Source: CAD feature listing. Evaluate the final solid. Frame: model axes, mm. Face numbers are marked on the shaded views. Coordinates: 2 decimals unless noted, no trailing zeros. Order: outer loops, then holes, each group sorted by start corner. A loop starts at its lowest first (then second) coordinate and runs counter-clockwise, first axis right, second up.
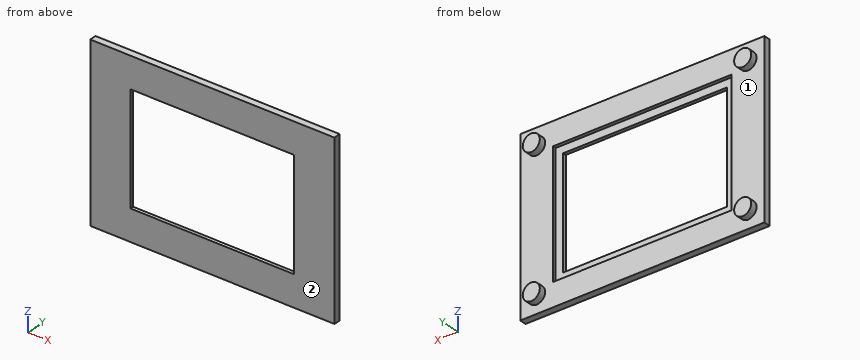
```python
from build123d import *

# Parameters (mm, degrees)
SKETCH1_W           = 35.8
SKETCH1_H           = 25
SKETCH1_W_2         = 24
SKETCH1_H_2         = 16
BOSS_EXTRUDE1_DEPTH = 1
SKETCH2_W           = 26.2
SKETCH2_H           = 18.2
CUT_EXTRUDE1_DEPTH  = 0.5
SKETCH4_R           = 1.25
BOSS_EXTRUDE2_DEPTH = 1


with BuildPart() as part:
    # Sketch1 → Boss-Extrude1 (new body)
    with BuildSketch(Plane(origin=(0, 0, 0), x_dir=(1, 0, 0), z_dir=(0, 1, 0))):
        Rectangle(SKETCH1_W, SKETCH1_H)
        Rectangle(SKETCH1_W_2, SKETCH1_H_2, mode=Mode.SUBTRACT)
    extrude(amount=BOSS_EXTRUDE1_DEPTH)

    # Sketch2 → Cut-Extrude1 (cut)
    with BuildSketch(Plane(origin=(0, 1, 0), x_dir=(1, 0, 0), z_dir=(0, 1, 0))):
        Rectangle(SKETCH2_W, SKETCH2_H)
    extrude(amount=-CUT_EXTRUDE1_DEPTH, mode=Mode.SUBTRACT)

    # Sketch4 → Boss-Extrude2 (add)
    with BuildSketch(Plane(origin=(0, 1, 0), x_dir=(1, 0, 0), z_dir=(0, 1, 0))):
        with Locations((-15.5, 10)):
            Circle(SKETCH4_R)
        with Locations((-15.5, -10)):
            Circle(SKETCH4_R)
        with Locations((15.5, -10)):
            Circle(SKETCH4_R)
        with Locations((15.5, 10)):
            Circle(SKETCH4_R)
    extrude(amount=BOSS_EXTRUDE2_DEPTH)


solid = part.part
```
1. Section query C-C, the plane x = 15.5. Output: boundary loops of the cut face in (y, z).
2. Draft query along X for the marked faces 1 and 2. Return one class per face: +X half, -X half, draft (parallel to the pull), parting line (faces both ways), or undercut.
3. Material intervals for line 1 along Z through (x, y) = (10, 0.6); line 2 along X through (y, z) = (0.75, 7.75); line 3 along X through (y, z) = (0.4, -7), sorted ascending.
4. Contact query for flat-ended pins moving along their axis: P1, Ø2, axis at x = -12, z = -7, coming from the +Y side; P2, Ø14.5, axis at x = -6.5, z = -4, coming from the +Y side; P3, Ø10, axis at x = 4, z = 1.5, coming from the +Y side. Output: stop coordinate, or through.
5. Section query B-B, the plane x = -5. Output: boundary loops of the cut face in (y, z).
6. Section query A-A, the plane z = -2.75. Output: boundary loops of the cut face in (x, y).
7. Section query D-D, the plane y = 1.35. Output: boundary loops of the cut face in (x, z), plus the area to 3 significant figures.
Answer key:
1. outline: (0, -12.5) - (1, -12.5) - (1, -11.25) - (2, -11.25) - (2, -8.75) - (1, -8.75) - (1, 8.75) - (2, 8.75) - (2, 11.25) - (1, 11.25) - (1, 12.5) - (0, 12.5) - close
2. face 1: undercut
2. face 2: draft
3. line 1: z = -12.5 to -9.1, 9.1 to 12.5
3. line 2: x = -17.9 to -13.1, 13.1 to 17.9
3. line 3: x = -17.9 to -12, 12 to 17.9
4. P1: stops at y = 0.5
4. P2: stops at y = 1
4. P3: passes through
5. outline: (0, -12.5) - (1, -12.5) - (1, -9.1) - (0.5, -9.1) - (0.5, -8) - (0, -8) - close; (0, 8) - (0.5, 8) - (0.5, 9.1) - (1, 9.1) - (1, 12.5) - (0, 12.5) - close
6. outline: (-17.9, 0) - (-12, 0) - (-12, 0.5) - (-13.1, 0.5) - (-13.1, 1) - (-17.9, 1) - close; (12, 0) - (17.9, 0) - (17.9, 1) - (13.1, 1) - (13.1, 0.5) - (12, 0.5) - close
7. outline: circle Ø2.5 at (-15.5, -10); circle Ø2.5 at (-15.5, 10); circle Ø2.5 at (15.5, -10); circle Ø2.5 at (15.5, 10)
7. area: 19.6 mm2
